Can you work these out from the model? Positions are in its coordinate system, mm. A direction names the side the tool comes from. Round coordinates to 2 decimals unless told otherwise and drop trailing zeros. Write each loop counter-clockwise with the first axis right and the second up, starting at its lowest first coordinate (ties: lowest second). Pieces come first, ordered by that corner, then holes.
Q1. We'd pull the mould along Y, two halves only. Please class faces 4 (the flat face through (40.6, 18, 5)), 5 (the cylindrical face through (-17.17, -2.87, 5.07)), 6 (the flat face through (-58, 25, 5)): +Y half, -Y half, draft (parallel to the pull), parting line (faces both ways), or undercut.
Q2. If we section it at B-B (x = -24): Please give me the cut outline in (y, z).
Q3. For faces 1 (the flat face through (-1, -25, 5)), 2 (the flat face through (-50.6, 17, 5)), 3 (the flat face through (-50.6, -17, 5)), which set-ups out of +Z, -Z, +X, -X, +Y, -Y let a thin tool reach every point of the face, with its end or its side?
Q4. If we section it at A-A (y = 0): Please give me the cut outline in (x, z), plus the area to 3 significant figures.
Q5. I'm going to push flat-ended pins straight in: pin 1 Ø9 at (x, y) = (-24.1, 0) entering from -Z; pin 2 Ø3 at (x, z) = (-45, 6.5) entering from +Y. Where does each tip first touch, or does it pass through?
Q6. If we section it at D-D (y = -13.5): Please give me the cut outline in (x, z), plus the area to 3 significant figures.
Q7. If we section it at C-C (z = 1.5): Please give me the cut outline in (x, y), plus the area to 3 significant figures.
Q8. Please list where these lines run through material, in increasing order: line 1 along X through (y, z) = (-23, 6.75); line 2 along X through (y, z) = (-0.5, 8.75); line 3 along Y through (x, z) = (-24.1, 6.5).
Autodesk Inventor part; units mm, degrees
ref_plane "YZ Plane" through (0, 0, 0) normal (1, 0, 0) x (0, 1, 0)
ref_plane "XZ Plane" through (0, 0, 0) normal (0, 1, 0) x (-1, 0, 0)
ref_plane "XY Plane" through (0, 0, 0) normal (0, 0, 1) x (1, 0, 0)
sketch "Sketch1" plane through (0, 0, 0) normal (0, 0, 1) x (1, 0, 0)
  line L0 (65.5, 25) -> (-65.5, 25)
  line L1 (-65.5, 25) -> (-65.5, -25)
  line L2 (-65.5, -25) -> (65.5, -25)
  line L3 (65.5, -25) -> (65.5, 25)
  line L4 (65.5, 25) -> (-65.5, -25) construction
  line L5 (-65.5, 25) -> (65.5, -25) construction
  line L6 (0, 0) -> (-24.1, 0)
  line L7 (0, 0) -> (24.1, 0)
  circle A0 centre (-24.1, 0) radius 7.5
  circle A1 centre (24.1, 0) radius 7.5
  dimension "d0" = 131
  dimension "d1" = 50
  dimension "d2" = 24.1
  dimension "d3" = 24.1
  dimension "d4" = 15
  dimension "d5" = 15
extrude "Extrusion1" add sketch "Sketch1" along normal blind 10
sketch "Sketch2" plane through (0, 0, 10) normal (0, 0, 1) x (1, 0, 0)
  circle A0 centre (24.1, 0) radius 7.5
  circle A1 centre (-24.1, 0) radius 7.5
  line L0 (65.5, 25) -> (-65.5, 25)
  line L1 (-65.5, 25) -> (-65.5, -25)
  line L2 (-65.5, -25) -> (65.5, -25)
  line L3 (65.5, -25) -> (65.5, 25)
  line L4 (-40.6, 25) -> (-40.6, 10)
  line L5 (-40.6, 10) -> (-50.6, 10)
  line L6 (-50.6, 10) -> (-50.6, 25)
  line L7 (-40.6, -25) -> (-40.6, -10)
  line L8 (-40.6, -10) -> (-50.6, -10)
  line L9 (-50.6, -10) -> (-50.6, -25)
  line L10 (40.6, 25) -> (40.6, 10)
  line L11 (40.6, 10) -> (50.6, 10)
  line L12 (50.6, 10) -> (50.6, 25)
  line L13 (40.6, -25) -> (40.6, -10)
  line L14 (40.6, -10) -> (50.6, -10)
  line L15 (50.6, -10) -> (50.6, -25)
  point P0 (0, 0)
  dimension "d10" = 15
  dimension "d12" = 15
  dimension "d14" = 15
  dimension "d16" = 15
sketch "Sketch3" plane through (0, 0, 10) normal (0, 0, 1) x (1, 0, 0)
  circle A0 centre (24.1, 0) radius 7.5
  circle A1 centre (-24.1, 0) radius 7.5
  line L0 (65.5, 25) -> (-65.5, 25)
  line L1 (-65.5, 25) -> (-65.5, -25)
  line L2 (-65.5, -25) -> (65.5, -25)
  line L3 (65.5, -25) -> (65.5, 25)
  point P0 (0, 0)
extrude "Extrusion2" cut sketch "Sketch3" against normal blind 10
extrude "Extrusion3" add sketch "Sketch2" against normal blind 10 contours L3 L2 L15 L14 L13 L7 L8 L9 L1 L0 L6 L5 L4 L10 L11 L12
properties part number "prepazka"
A:
1. face 4: draft
1. face 5: undercut
1. face 6: +Y half
2. outline: (-25, 0) - (-7.5, 0) - (-7.5, 10) - (-25, 10) - close; (7.5, 0) - (25, 0) - (25, 10) - (7.5, 10) - close
3. face 1: +Z, -Z, +X, -X, -Y
3. face 2: +Z, -Z, +Y
3. face 3: +Z, -Z, -Y
4. outline: (-65.5, 0) - (-31.6, 0) - (-31.6, 10) - (-65.5, 10) - close; (-16.6, 0) - (16.6, 0) - (16.6, 10) - (-16.6, 10) - close; (31.6, 0) - (65.5, 0) - (65.5, 10) - (31.6, 10) - close
4. area: 1,010 mm2
5. pin 1: passes through
5. pin 2: stops at y = 10
6. outline: (-65.5, 0) - (-50.6, 0) - (-50.6, 10) - (-65.5, 10) - close; (-40.6, 0) - (40.6, 0) - (40.6, 10) - (-40.6, 10) - close; (50.6, 0) - (65.5, 0) - (65.5, 10) - (50.6, 10) - close
6. area: 1,110 mm2
7. outline: (-65.5, -25) - (-50.6, -25) - (-50.6, -10) - (-40.6, -10) - (-40.6, -25) - (40.6, -25) - (40.6, -10) - (50.6, -10) - (50.6, -25) - (65.5, -25) - (65.5, 25) - (50.6, 25) - (50.6, 10) - (40.6, 10) - (40.6, 25) - (-40.6, 25) - (-40.6, 10) - (-50.6, 10) - (-50.6, 25) - (-65.5, 25) - close; hole circle Ø15 at (-24.1, 0); hole circle Ø15 at (24.1, 0)
7. area: 5,600 mm2
8. line 1: x = -65.5 to -50.6, -40.6 to 40.6, 50.6 to 65.5
8. line 2: x = -65.5 to -31.58, -16.62 to 16.62, 31.58 to 65.5
8. line 3: y = -25 to -7.5, 7.5 to 25
